from build123d import *

# Parameters (mm, degrees)
F2_R     = 24.5
F3_DEPTH = 14.540077
F4_R     = 3.5
F5_DEPTH = 5.540077


with BuildPart() as f1:
    # F0 (on Front) → F1 (revolve)
    with BuildSketch(Plane.XZ):
        with BuildLine():
            Line((16.65759, 20.249971), (8.641342, 20.249971))
            ThreePointArc((8.641342, 20.249971), (5.963574, 18.780897), (5.763815, 15.733158))
            Line((5.763815, 15.733158), (11.118513, 4.249971))
            Line((11.118513, 4.249971), (11.118513, -8.750029))
            Line((11.118513, -8.750029), (2.118513, -8.750029))
            Line((2.118513, -8.750029), (2.118513, -34.750036))
            Line((2.118513, -34.750036), (16.65759, -34.750036))
            Line((16.65759, -34.750036), (16.65759, 4.249971))
            Line((16.65759, 4.249971), (16.65759, 20.249971))
        make_face()
    revolve(axis=Axis((9.388052, 0, -34.750036), (1, 0, 0)))

    # F2 (on face) → F3 (cut, through all)
    with BuildSketch(Plane(origin=(2.118513, 0, 0), x_dir=(0, -1, 0), z_dir=(-1, 0, 0))):
        with Locations((0, -34.750036)):
            Circle(F2_R)
    extrude(amount=-F3_DEPTH, mode=Mode.SUBTRACT)

    # F4 (on face) → F5 (cut, through all)
    with BuildSketch(Plane(origin=(11.118513, 0, 0), x_dir=(0, -1, 0), z_dir=(-1, 0, 0))):
        with Locations((0, -1.250036)):
            Circle(F4_R)
        with Locations((-29.011851, -18.000036)):
            Circle(F4_R)
        with Locations((-29.011851, -51.500036)):
            Circle(F4_R)
        with Locations((0, -68.250036)):
            Circle(F4_R)
        with Locations((29.011851, -51.500036)):
            Circle(F4_R)
        with Locations((29.011851, -18.000036)):
            Circle(F4_R)
    extrude(amount=-F5_DEPTH, mode=Mode.SUBTRACT)


solid = f1.part
Geometry check sheet. Reference: the model listing, model coordinates, mm. A direction names the side the tool comes from. Round coordinates to 2 decimals unless told otherwise and drop trailing zeros. Write each loop counter-clockwise with the first axis right and the second up, starting at its lowest first coordinate (ties: lowest second). Pieces come first, ordered by that corner, then holes.
Item 1: Mould release check, pull along X, two halves, no side actions. Record for faces 1 (the face through (11.119, 25, -27)), 2 (the face through (16.658, -1, -10)), 3 (the face through (13.849, 0.759, -71.667)): +X half, -X half, draft (parallel to the pull), parting line (faces both ways), or undercut.
Determined:
face 1: -X half
face 2: +X half
face 3: draft
Item 2: Access from +Z, -Z, +X, -X, +Y, -Y to the whole of each face (thin tool, end or side, straight path). Record for faces 4 (the face through (6.556, 9.958, -10.733)), 5 (the face through (9.29, 3.19, -10.46)).
Determined:
face 4: -X
face 5: +X, -X
Item 3: Section check A-A (y = 0). Record the boundary of the cut face in (x, z) (3 decimals), plus the area to 3 significant figures.
Determined:
outline: (2.119, -60.75) - (11.119, -60.75) - (11.119, -64.75) - (16.658, -64.75) - (16.658, -59.25) - (2.119, -59.25) - close; (2.119, -10.25) - (16.658, -10.25) - (16.658, -4.75) - (11.119, -4.75) - (11.119, -8.75) - (2.119, -8.75) - close; (5.764, -85.233) arc R3.175 ccw to (8.641, -89.75) - (16.658, -89.75) - (16.658, -71.75) - (11.119, -71.75) - (11.119, -73.75) - close; (5.764, 15.733) - (11.119, 4.25) - (11.119, 2.25) - (16.658, 2.25) - (16.658, 20.25) - (8.641, 20.25) arc R3.175 ccw to start
area: 395 mm2
Item 4: Go/stop test with flat-tipped pins: pin 1 Ø8 at (x, y) = (4, 31.5) entering from +Z; pin 2 Ø3 at (x, z) = (10.5, -15) entering from +Y; pin 3 Ø9 at (y, z) = (-29.01, -51.5) entering from -X; pin 4 Ø8 at (y, z) = (-29.01, -18) entering from +X. Record where each tip stops, or that it passes through.
Determined:
pin 1: stops at z = 11.54
pin 2: stops at y = 51.88
pin 3: stops at x = 11.12
pin 4: stops at x = 16.66
Item 5: Material ranges on line 1 along Z through (x, y) = (14.7, 0); line 2 along Y through (x, z) = (8.5, -44); line 3 along Y through (x, z) = (7, -53), recorded low to high.
Determined:
line 1: z = -89.75 to -71.75, -64.75 to -59.25, -10.25 to -4.75, 2.25 to 20.25
line 2: y = -54.21 to -43.65, -24.3 to -22.69, 22.69 to 24.3, 43.65 to 54.21
line 3: y = -51.4 to -44.21, -18.52 to -16.35, 16.35 to 18.52, 44.21 to 51.4
